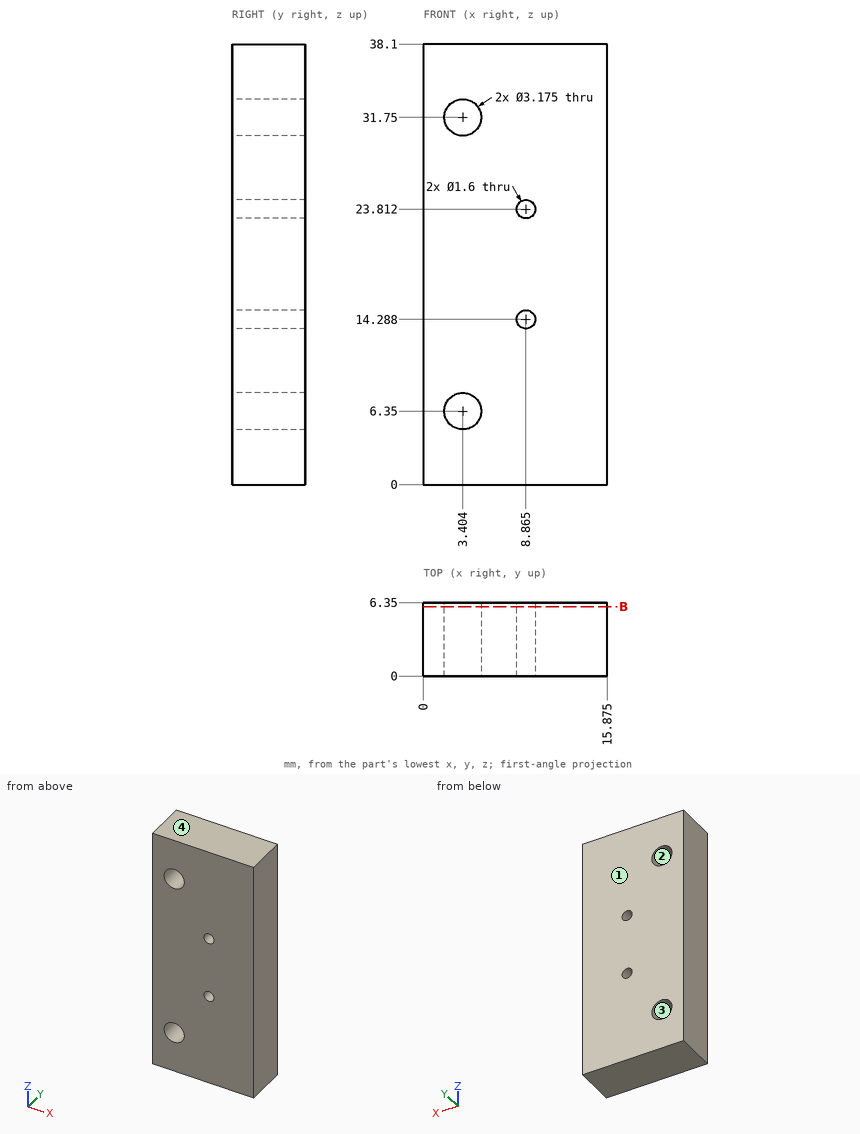
Design review of the part shown in the three views and the two pictorial views. Dimensions are in mm from the part's minimum x, y and z. Round coordinates to 2 decimals unless told otherwise and drop trailing zeros. Use CSV: the item, a comma, the result in double quotes.
(1) For line 1 (Z direction, x = 2.5, y = 3.5) (1 decimal); line 2 (X direction, y = 2.25, z = 32) (1 decimal); line 3 (X direction, y = 2.5, z = 14) (1 decimal), list the stretches that pass through material, from the lowest coordinate up.
Working result:
line 1,"z = 0 to 5, 7.7 to 30.4, 33.1 to 38.1"
line 2,"x = 0 to 1.8, 5 to 15.9"
line 3,"x = 0 to 8.1, 9.6 to 15.9"
(2) Take a section at B-B, the plane y = 6. State how many separate pieces and enclosed holes the cut face has, plus the area to 3 significant figures.
Working result:
separate pieces,"1"
enclosed holes,"4"
area,"585 mm^2"
(3) The part is to be moulded in two halves that separate along Z. For the marked faces 1, 2, 3 and 4, say which applies: pulls with the +Z half, pulls with the -Z half, needs draft (parallel to the pull), parting line crosses it, or undercut.
Working result:
face 1,"needs draft"
face 2,"undercut"
face 3,"undercut"
face 4,"pulls with the +Z half"
(4) Clearance check with a flat-ended pin moving along its axis: P1, Ø2.5, axis at x = 3.4, z = 31.75, coming from the -Y side. State where the tip first meets the part, or that it passes through.
Working result:
P1,"passes through"
